```python
from build123d import *

# Parameters (mm, degrees)
F0_R     = 14
F1_DEPTH = 244
F2_W     = 60
F2_H     = 40
F3_DEPTH = 80
F4_R     = 5
F6_DEPTH = 40
F8_DEPTH = 35


with BuildPart() as f1:
    # F0 (on Top) → F1 (new body)
    with BuildSketch(Plane.XY):
        Circle(F0_R)
    extrude(amount=F1_DEPTH)

    # F2 (on Top) → F3 (join)
    with BuildSketch(Plane.XY):
        Rectangle(F2_W, F2_H)
    extrude(amount=-F3_DEPTH)

    # F4
    f4_edges = [f1.edges().sort_by_distance(p)[0] for p in [
        (30, -20, -40),
        (30, 20, -40),
        (-30, -20, -40),
        (-30, 20, -40),
    ]]
    fillet(f4_edges, radius=F4_R)

    # F5 (on Front) → F6 (cut, symmetric)
    with BuildSketch(Plane.XZ):
        with BuildLine():
            Line((-30, 0), (-30, -90))
            Line((-30, -90), (30, -90))
            Line((30, -90), (30, 0))
            ThreePointArc((30, 0), (23.0927925952, -40.9972362717), (4.0380677708, -77.9485604417))
            ThreePointArc((4.0380677708, -77.9485604417), (2.2646410082, -79.4577349746), (0, -80))
            ThreePointArc((0, -80), (-3.4564291769, -78.6129070491), (-4.9951029351, -75.2212389381))
            ThreePointArc((-4.9951029351, -75.2212389381), (-10.5871286649, -45.3841026089), (-24.2616371934, -18.2818283023))
            ThreePointArc((-24.2616371934, -18.2818283023), (-28.5317146762, -9.5806322048), (-30, 0))
        make_face()
    extrude(amount=F6_DEPTH, both=True, mode=Mode.SUBTRACT)

    # F7 (on Right) → F8 (cut, symmetric)
    with BuildSketch(Plane.YZ):
        with BuildLine():
            Line((13, -80), (13, -50))
            add(Edge.make_bspline(
                [(13, -50), (13, -20), (0, -20), (-13, -20), (-13, -50)],
                knots=[1.5707963268, 1.5707963268, 1.5707963268, 3.1415926536, 3.1415926536, 4.7123889804, 4.7123889804, 4.7123889804], degree=2, weights=[1, 0.7071067812, 1, 0.7071067812, 1]))
            Line((-13, -50), (-13, -80))
            Line((-13, -80), (13, -80))
        make_face()
    extrude(amount=F8_DEPTH, both=True, mode=Mode.SUBTRACT)


solid = f1.part
```
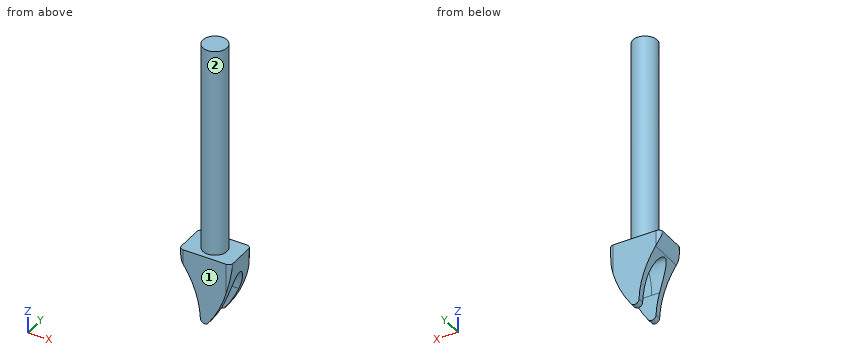
Input: part model. Units: mm. Frame: model coordinates. Face numbers are marked on the shaded views. A direction names the side the tool comes from. Round coordinates to 2 decimals unless told otherwise and drop trailing zeros. Write each loop counter-clockwise with the first axis right and the second up, starting at its lowest first coordinate (ties: lowest second). Pieces come first, ordered by that corner, then holes. Notation, with made-up numbers: (-34, 82.25) - (-4, 82.25) arc R12 ccw to (-4, 88.25) - close; hole circle Ø2 at (-14, 32). An arc over 180 degrees is marked (long way). Write item = value, one per line.
(1) Section query B-B on z = 221.5. Output: boundary loops of the cut face in (x, y), then the cut area to 3 significant figures.
Geometry check:
outline = circle Ø28 at (0, 0)
area = 616 mm^2
(2) Material intervals for probe 1 along Y at (x, z) = (6, -53); probe 2 along X at (y, z) = (-1, 190.5); probe 3 along Z at (x, y) = (-4, 17), sorted ascending.
Geometry check:
probe_1 = -20 to -13, 13 to 20
probe_2 = -13.96 to 13.96
probe_3 = -78 to 0
(3) Contact query for flat-ended pins moving along their axis: pin 1 Ø8 at (x, z) = (19, 195.5) entering from +Y; pin 2 Ø12 at (x, y) = (-13.5, 12.5) entering from +Z; pin 3 Ø10 at (y, z) = (1, 29) entering from -X; pin 4 Ø4 at (y, z) = (9.5, 10.5) entering from -X. Output: stop coordinate, or through.
Geometry check:
pin_1 = through
pin_2 = 244
pin_3 = -14
pin_4 = -11.82
(4) Section query A-A on z = -53. Output: boundary loops of the cut face in (x, y), then the cut area to 3 significant figures.
Geometry check:
outline = (-8.32, -20) - (18.45, -20) - (18.45, -13) - (-8.32, -13) - close; (-8.32, 13) - (18.45, 13) - (18.45, 20) - (-8.32, 20) - close
area = 375 mm^2
(5) Access query for the marked faces 1 and 2. Directions: +Z, -Z, +X, -X, +Y, -Y. A direction counts if a zero-diameter tool reaches every point of the face in a straight line with its end or side. Return the directions, or none.
Geometry check:
face_1 = +Z, -Z, +X, -X, -Y
face_2 = +Z
